from build123d import *

# Parameters (mm, degrees)
F0_W          = 1.75
F0_H          = 1.5
F0_W_2        = 2.25
F0_H_2        = 4.5
F0_H_3        = 2.7
F2_DEPTH      = 3.25
F3_ANGLE_BACK = 35
F3_ANGLE      = 70
F4_DEPTH      = 12.5
F5_DEPTH      = 5
F6_START      = 3.25
F6_DEPTH      = 4.351
F7_DEPTH      = 7.601


with BuildPart() as f1:
    # F0 (on Front) → F1 (revolve)
    with BuildSketch(Plane.XZ):
        Polygon((-1.75, 0), (-7.6, 0), (-7.6, -1.5), (-5.1, -1.5), (-2.85, -1.5), (-1.75, -1.5), align=None)
        with BuildLine():
            ThreePointArc((0, 2), (-3.9293765409, 1.4916308553), (-7.6, 0))
            Line((-7.6, 0), (-1.75, 0))
            Line((-1.75, 0), (0, 0))
            Line((0, 0), (0, 2))
        make_face()
        with Locations((-0.875, -0.75)):
            Rectangle(F0_W, F0_H)
    revolve(axis=Axis((0, 0, 1), (0, 0, 1)))

    # F0 (on Front) → F2 (join, symmetric)
    with BuildSketch(Plane.XZ):
        with Locations((-3.975, -3.75)):
            Rectangle(F0_W_2, F0_H_2)
        with Locations((-3.975, -7.35)):
            Rectangle(F0_W_2, F0_H_3)
        with Locations((3.975, -7.35)):
            Rectangle(F0_W_2, F0_H_3)
        with Locations((3.975, -3.75)):
            Rectangle(F0_W_2, F0_H_2)
    extrude(amount=F2_DEPTH, both=True)

    # F0 (on Front) → F3 (revolve)
    with BuildSketch(Plane.XZ, mode=Mode.PRIVATE) as f3_sk:
        Polygon((-5.1, -8.7), (-5.1, -6), (-7.35, -6), (-6.15, -8.7), align=None)
        Polygon((7.35, -6), (5.1, -6), (5.1, -8.7), (6.15, -8.7), align=None)
    revolve(f3_sk.sketch.rotate(Axis((0, 0, 1), (0, 0, 1)), -F3_ANGLE_BACK), axis=Axis((0, 0, 1), (0, 0, 1)), revolution_arc=F3_ANGLE)

    # F0 (on Front) → F4 (cut, symmetric)
    with BuildSketch(Plane.XZ):
        with Locations((-0.875, -0.75)):
            Rectangle(F0_W, F0_H)
        with Locations((0.875, -0.75)):
            Rectangle(F0_W, F0_H)
    extrude(amount=F4_DEPTH, both=True, mode=Mode.SUBTRACT)

    # F0 (on Front) → F5 (join, symmetric)
    with BuildSketch(Plane.XZ):
        Polygon((0, -1.5), (-1.75, -1.5), (-1.75, -2.85), (1.75, -2.85), (1.75, -1.5), align=None)
        with Locations((-0.875, -0.75)):
            Rectangle(F0_W, F0_H)
        with Locations((0.875, -0.75)):
            Rectangle(F0_W, F0_H)
    extrude(amount=F5_DEPTH, both=True)

    # F0 (on Front) → F6 (cut)
    with BuildSketch(Plane.XZ.offset(F6_START)):
        Polygon((-5.1, -8.7), (-5.1, -6), (-7.35, -6), (-6.15, -8.7), align=None)
        with Locations((-3.975, -7.35)):
            Rectangle(F0_W_2, F0_H_3)
        with Locations((3.975, -7.35)):
            Rectangle(F0_W_2, F0_H_3)
        Polygon((7.35, -6), (5.1, -6), (5.1, -8.7), (6.15, -8.7), align=None)
    extrude(amount=F6_DEPTH, mode=Mode.SUBTRACT)

    # F0 (on Front) → F7 (cut, through all)
    with BuildSketch(Plane.XZ):
        Polygon((7.35, -6), (5.1, -6), (5.1, -8.7), (6.15, -8.7), align=None)
        Polygon((-5.1, -8.7), (-5.1, -6), (-7.35, -6), (-6.15, -8.7), align=None)
        Polygon((0, -1.5), (-1.75, -1.5), (-1.75, -2.85), (1.75, -2.85), (1.75, -1.5), align=None)
        with Locations((3.975, -3.75)):
            Rectangle(F0_W_2, F0_H_2)
        with Locations((3.975, -7.35)):
            Rectangle(F0_W_2, F0_H_3)
        with Locations((-3.975, -3.75)):
            Rectangle(F0_W_2, F0_H_2)
        with Locations((-3.975, -7.35)):
            Rectangle(F0_W_2, F0_H_3)
        with BuildLine():
            ThreePointArc((7.6, 0), (3.9293765409, 1.4916308553), (0, 2))
            Line((0, 2), (0, 0))
            Line((0, 0), (1.75, 0))
            Line((1.75, 0), (7.6, 0))
        make_face()
        with BuildLine():
            ThreePointArc((0, 2), (-3.9293765409, 1.4916308553), (-7.6, 0))
            Line((-7.6, 0), (-1.75, 0))
            Line((-1.75, 0), (0, 0))
            Line((0, 0), (0, 2))
        make_face()
        Polygon((-1.75, 0), (-7.6, 0), (-7.6, -1.5), (-5.1, -1.5), (-2.85, -1.5), (-1.75, -1.5), align=None)
        Polygon((7.6, -1.5), (7.6, 0), (1.75, 0), (1.75, -1.5), (2.85, -1.5), (5.1, -1.5), align=None)
        with Locations((-0.875, -0.75)):
            Rectangle(F0_W, F0_H)
        with Locations((0.875, -0.75)):
            Rectangle(F0_W, F0_H)
    extrude(amount=-F7_DEPTH, mode=Mode.SUBTRACT)


solid = f1.part
Verification items for the finished model (mm, model axes). A direction names the side the tool comes from. Coordinates: 2 decimals unless noted, no trailing zeros. Write each loop counter-clockwise with the first axis right and the second up, starting at its lowest first coordinate (ties: lowest second). Pieces come first, ordered by that corner, then holes. Notation, with made-up numbers: (53, -9.5) - (58, -9.5) arc R25 ccw to (58, 29.5) - close; hole circle Ø2 at (-33.75, -13). An arc over 180 degrees is marked (long way). Answer as a JSON object with one key per item and string values.
(1) Thickness scan on line 1 along X through (y, z) = (-1.75, -3); line 2 along Y through (x, z) = (-5, -6.5); line 3 along X through (y, z) = (-2.5, -7.25). Record the ranges inside material, lowest first.
Report:
{"line 1": "-5.1 to -2.85, 2.85 to 5.1", "line 2": "-3.25 to 0", "line 3": "-6.32 to -2.85, 2.85 to 6.32"}
(2) Mould release check, pull along Z, two halves, no side actions. Record for faces 1 (the flat face through (-1.75, -3, -2)), 2 (the flat face through (-5, -2, -8.7)), 3 (the flat face through (-4, -4, -1.5)): pulls with the +Z half, pulls with the -Z half, needs draft (parallel to the pull), parting line crosses it, or undercut.
Report:
{"face 1": "needs draft", "face 2": "pulls with the -Z half", "face 3": "undercut"}
(3) Cross-section at B-B on z = -2.25. Record the cut outline in (x, y).
Report:
{"outline": "(-5.1, -3.25) - (-2.85, -3.25) - (-2.85, 0) - (-5.1, 0) - close; (-1.75, -5) - (1.75, -5) - (1.75, 0) - (-1.75, 0) - close; (2.85, -3.25) - (5.1, -3.25) - (5.1, 0) - (2.85, 0) - close"}
(4) Gauge pin test, flat ends, axial feed: pin 1 Ø1 at (x, y) = (1.5, -2.5) entering from -Z; pin 2 Ø1 at (y, z) = (-1.5, -3.5) entering from -X; pin 3 Ø1.5 at (y, z) = (-2, -2.5) entering from +X. Record the tip position at first contact, or that the pin passes through.
Report:
{"pin 1": "z = -2.85", "pin 2": "x = -5.1", "pin 3": "x = 5.1"}
(5) Cross-section at D-D on x = -0.75. Record the cut outline in (y, z), plus the area to 3 significant figures.
Report:
{"outline": "(-7.56, 0) - (-5, 0) - (-5, -2.85) - (0, -2.85) - (0, 1.98) arc R15.42 ccw to start", "area": "24.4 mm^2"}
(6) Tool access check on faces 4 (the flat face through (-6, -1, -6)), 5 (the flat face through (0, -5, -1)), 6 (the flat face through (4, -3.25, -5)), 7 (the flat face through (2.85, -2, -5)). Record the directions out of +Z, -Z, +X, -X, +Y, -Y that give a thin tool (end or side, any length) a straight path to the whole face; none if there is none.
Report:
{"face 4": "-X, +Y, -Y", "face 5": "-Z, -Y", "face 6": "-Z, +X, -Y", "face 7": "-Z, +Y, -Y"}
(7) Cross-section at C-C on y = -4. Record the cut outline in (x, z).
Report:
{"outline": "(-6.46, -1.5) - (-1.75, -1.5) - (-1.75, -2.85) - (1.75, -2.85) - (1.75, -1.5) - (6.46, -1.5) - (6.46, 0) arc R14.91 ccw to (-6.46, 0) - close"}
(8) Cross-section at A-A on z = -4.75. Record the cut outline in (x, y).
Report:
{"outline": "(-5.1, -3.25) - (-2.85, -3.25) - (-2.85, 0) - (-5.1, 0) - close; (2.85, -3.25) - (5.1, -3.25) - (5.1, 0) - (2.85, 0) - close"}
